```python
from build123d import *

# Parameters (mm, degrees)
SKETCH2_R         = 30
ACRYLICBASE_DEPTH = 1
SKETCH3_W         = 5
SKETCH3_H         = 26
WHEELS_DEPTH      = 43.473521163
SKETCH4_R         = 2.15265
HOLES_DEPTH       = 43.473521163
FLATSIDES_DEPTH   = 43.473521163
RELIEFS_R         = 2


with BuildPart() as part:
    # Sketch2 → AcrylicBase (new, symmetric)
    with BuildSketch(Plane(origin=(0, 0, 0), x_dir=(1, 0, 0), z_dir=(0, 1, 0))):
        with Locations(Location((0, 0, 0), (0, 0, 270))):
            Circle(SKETCH2_R)
    extrude(amount=ACRYLICBASE_DEPTH, both=True)

    # Sketch3 → wheels (cut, through all)
    with BuildSketch(Plane(origin=(0, 1, 0), x_dir=(1, 0, 0), z_dir=(0, 1, 0))):
        with Locations((-20.657104633, 0)):
            Rectangle(SKETCH3_W, SKETCH3_H)
        with Locations((20.657104633, 0)):
            Rectangle(SKETCH3_W, SKETCH3_H)
    extrude(amount=-WHEELS_DEPTH, mode=Mode.SUBTRACT)

    # Sketch4 → holes (cut, through all)
    with BuildSketch(Plane(origin=(0, 1, 0), x_dir=(1, 0, 0), z_dir=(0, 1, 0))):
        with Locations(Location((-17.5, 17.5, 0), (0, 0, 270))):
            Circle(SKETCH4_R)
        with Locations(Location((-17.5, -17.5, 0), (0, 0, 270))):
            Circle(SKETCH4_R)
        with Locations(Location((17.5, -17.5, 0), (0, 0, 270))):
            Circle(SKETCH4_R)
        with Locations(Location((17.5, 17.5, 0), (0, 0, 270))):
            Circle(SKETCH4_R)
    extrude(amount=-HOLES_DEPTH, mode=Mode.SUBTRACT)

    # Sketch5 → flatSides (cut, through all)
    with BuildSketch(Plane(origin=(0, 1, 0), x_dir=(1, 0, 0), z_dir=(0, 1, 0))):
        with BuildLine():
            ThreePointArc((-25.657104633, 15.547121337), (-30, 0), (-25.657104633, -15.547121337))
            Line((-25.657104633, -15.547121337), (-25.657104633, 15.547121337))
        make_face()
        with BuildLine():
            Line((25.657104633, 15.547121337), (25.657104633, -15.547121337))
            ThreePointArc((25.657104633, -15.547121337), (28.893884638, -8.071148029), (30, 0))
            ThreePointArc((30, 0), (28.893884638, 8.071148029), (25.657104633, 15.547121337))
        make_face()
    extrude(amount=-FLATSIDES_DEPTH, mode=Mode.SUBTRACT)

    # reliefs
    reliefs_edges = [part.edges().sort_by_distance(p)[0] for p in [
        (-18.157104633, 0, -13),
        (-18.157104633, 0, 13),
        (23.157104633, 0, -13),
        (23.157104633, 0, 13),
        (18.157104633, 0, 13),
        (18.157104633, 0, -13),
        (-25.657104633, 0, 15.547121337),
        (-25.657104633, 0, -15.547121337),
        (25.657104633, 0, 15.547121337),
        (25.657104633, 0, -15.547121337),
        (-23.157104633, 0, 13),
        (-23.157104633, 0, -13),
    ]]
    fillet(reliefs_edges, radius=RELIEFS_R)


solid = part.part
```
For this review, take the finished solid that the model builds, in its own axes (mm). A direction names the side the tool comes from. Round coordinates to 2 decimals unless told otherwise and drop trailing zeros. Write each loop counter-clockwise with the first axis right and the second up, starting at its lowest first coordinate (ties: lowest second). Pieces come first, ordered by that corner, then holes. Notation, with made-up numbers: (-26, -22) - (-14, -22) arc R14 cw to (-14, -9) - close; hole circle Ø3 at (18.25, 85). An arc over 180 degrees is marked (long way). Answer as a JSON object with one key per item and string values.
1. Tool access review of faces 4 (the face through (-18.73, -0.01, 12.4)), 5 (the face through (-25.657, 0, 0)): name each direction out of +Z, -Z, +X, -X, +Y, -Y from which nothing blocks a thin tool from reaching the whole face with its end or side.
Response values:
{"face 4": "+Y, -Y", "face 5": "+Z, -Z, -X, +Y, -Y"}
2. We need section A-A on z = 9.5. Give the boundary of the cut face in (x, y).
Response values:
{"outline": "(-25.66, -1) - (-23.16, -1) - (-23.16, 1) - (-25.66, 1) - close; (-18.16, -1) - (18.16, -1) - (18.16, 1) - (-18.16, 1) - close; (23.16, -1) - (25.66, -1) - (25.66, 1) - (23.16, 1) - close"}
3. Draft analysis for pull direction Z (two halves, no side actions). For faces 1 (the face through (0, 0, -30)), 2 (the face through (19.634, 0.014, -17.78)), 3 (the face through (0, 1, 0)), state which applies: +Z half, -Z half, draft (parallel to the pull), parting line (faces both ways), or undercut.
Response values:
{"face 1": "-Z half", "face 2": "undercut", "face 3": "draft"}
4. We need section C-C on x = -17.5. Give the boundary of the cut face in (y, z), then the cut area to 3 significant figures.
Response values:
{"outline": "(-1, -24.37) - (1, -24.37) - (1, -19.65) - (-1, -19.65) - close; (-1, -15.35) - (1, -15.35) - (1, 15.35) - (-1, 15.35) - close; (-1, 19.65) - (1, 19.65) - (1, 24.37) - (-1, 24.37) - close", "area": "80.2 mm2"}
5. For pin 1 Ø0.5 at (x, y) = (21, 0) entering from -Z; pin 2 Ø0.5 at (x, y) = (20.5, 0.5) entering from +Z; pin 3 Ø0.8 at (x, y) = (-21, 0) entering from -Z; pin 4 Ø2.5 at (x, z) = (-17.5, -17.5) entering from +Y, all flat-tipped, find the tip position at first contact; note any pin that passes through.
Response values:
{"pin 1": "stops at z = -21.67", "pin 2": "stops at z = 22.13", "pin 3": "stops at z = -21.81", "pin 4": "passes through"}
6. We need section B-B on y = 0.4. Give the boundary of the cut face in (x, z), then the cut area to 3 significant figures.
Response values:
{"outline": "(-25.66, -14.98) arc R2 ccw to (-25.35, -16.05) arc R30 ccw to (25.35, -16.05) arc R2 ccw to (25.66, -14.98) - (25.66, 14.98) arc R2 ccw to (25.35, 16.05) arc R30 ccw to (-25.35, 16.05) arc R2 ccw to (-25.66, 14.98) - close; hole (-23.16, -11) arc R2 ccw to (-21.16, -13) - (-20.16, -13) arc R2 ccw to (-18.16, -11) - (-18.16, 11) arc R2 ccw to (-20.16, 13) - (-21.16, 13) arc R2 ccw to (-23.16, 11) - close; hole circle Ø4.31 at (-17.5, -17.5); hole circle Ø4.31 at (-17.5, 17.5); hole circle Ø4.31 at (17.5, -17.5); hole circle Ø4.31 at (17.5, 17.5); hole (18.16, -11) arc R2 ccw to (20.16, -13) - (21.16, -13) arc R2 ccw to (23.16, -11) - (23.16, 11) arc R2 ccw to (21.16, 13) - (20.16, 13) arc R2 ccw to (18.16, 11) - close", "area": "2,330 mm2"}
7. We need section D-D on z = -24.5. Give the boundary of the cut face in (x, y).
Response values:
{"outline": "(-17.31, -1) - (17.31, -1) - (17.31, 1) - (-17.31, 1) - close"}
8. To check wall thickness, follow line 1 along X through (y, z) = (-0.1, -1); line 2 along X through (y, z) = (-0.4, 17.5); line 3 along Z through (x, y) = (-17, 0.65). State the ranges of each line that lie inside material, in increasing order.
Response values:
{"line 1": "x = -25.66 to -23.16, -18.16 to 18.16, 23.16 to 25.66", "line 2": "x = -24.37 to -19.65, -15.35 to 15.35, 19.65 to 24.37", "line 3": "z = -24.72 to -19.59, -15.41 to 15.41, 19.59 to 24.72"}
